```python
from build123d import *

# Parameters (mm, degrees)
SKETCH1_R           = 101.6
BOSS_EXTRUDE1_DEPTH = 25.4
CUT_EXTRUDE1_DEPTH  = 25.4
SKETCH3_R           = 12.7
CUT_EXTRUDE2_DEPTH  = 25.4


with BuildPart() as part:
    # Sketch1 → Boss-Extrude1 (new body)
    with BuildSketch(Plane(origin=(0, 0, 0), x_dir=(1, 0, 0), z_dir=(0, 1, 0))):
        with Locations(Location((0, 0, 0), (0, 0, 270))):
            Circle(SKETCH1_R)
    extrude(amount=BOSS_EXTRUDE1_DEPTH)

    # Sketch2 → Cut-Extrude1 (cut)
    with BuildSketch(Plane(origin=(0, 25.4, 0), x_dir=(1, 0, 0), z_dir=(0, 1, 0))):
        with BuildLine():
            Line((0, 91.44), (16.738974461, 91.44))
            ThreePointArc((16.738974461, 91.44), (20.64808073, 89.604270053), (21.73196517, 85.423814242))
            Line((21.73196517, 85.423814242), (16.01696517, 54.943814242))
            ThreePointArc((16.01696517, 54.943814242), (14.268244513, 51.970893731), (11.023974461, 50.8))
            Line((11.023974461, 50.8), (0, 50.8))
            Line((0, 50.8), (-11.023974461, 50.8))
            ThreePointArc((-11.023974461, 50.8), (-14.268244513, 51.970893731), (-16.01696517, 54.943814242))
            Line((-16.01696517, 54.943814242), (-21.73196517, 85.423814242))
            ThreePointArc((-21.73196517, 85.423814242), (-20.64808073, 89.604270053), (-16.738974461, 91.44))
            Line((-16.738974461, 91.44), (0, 91.44))
        make_face()
        with BuildLine():
            Line((38.26171821, 79.407476156), (23.047495859, 52.38491034))
            ThreePointArc((23.047495859, 52.38491034), (22.476137132, 48.983465131), (24.208756195, 46.001131903))
            Line((24.208756195, 46.001131903), (32.653610572, 38.91505771))
            Line((32.653610572, 38.91505771), (41.098464949, 31.828983518))
            ThreePointArc((41.098464949, 31.828983518), (44.336355977, 30.640563561), (47.586910188, 31.793896828))
            Line((47.586910188, 31.793896828), (71.557020524, 51.469400264))
            ThreePointArc((71.557020524, 51.469400264), (73.413862069, 55.368522696), (71.599297399, 59.287498497))
            Line((71.599297399, 59.287498497), (58.77649903, 70.047103879))
            Line((58.77649903, 70.047103879), (45.953700661, 80.806709261))
            ThreePointArc((45.953700661, 80.806709261), (41.77916706, 81.913183611), (38.26171821, 79.407476156))
        make_face()
        with BuildLine():
            Line((80.352318408, 36.23549746), (51.327777432, 25.314524697))
            ThreePointArc((51.327777432, 25.314524697), (48.703684419, 23.076128807), (48.113940777, 19.677822943))
            Line((48.113940777, 19.677822943), (50.028233853, 8.821327425))
            Line((50.028233853, 8.821327425), (51.942526929, -2.035168092))
            ThreePointArc((51.942526929, -2.035168092), (53.658993735, -5.026826831), (56.890411059, -6.232738262))
            Line((56.890411059, -6.232738262), (87.899750706, -6.568118115))
            ThreePointArc((87.899750706, -6.568118115), (91.828481442, -4.774771782), (92.957513347, -0.606282461))
            Line((92.957513347, -0.606282461), (90.050820935, 15.878389366))
            Line((90.050820935, 15.878389366), (87.144128524, 32.363061192))
            ThreePointArc((87.144128524, 32.363061192), (84.65747826, 35.894008194), (80.352318408, 36.23549746))
        make_face()
        with BuildLine():
            Line((84.845175807, -23.891473209), (55.5912215, -13.600808392))
            ThreePointArc((55.5912215, -13.600808392), (52.142236485, -13.628784649), (49.506077743, -15.852958066))
            Line((49.506077743, -15.852958066), (43.994090512, -25.4))
            Line((43.994090512, -25.4), (38.482103282, -34.947041934))
            ThreePointArc((38.482103282, -34.947041934), (37.873991971, -38.342109081), (39.574256329, -41.34300585))
            Line((39.574256329, -41.34300585), (63.113210637, -61.532341033))
            ThreePointArc((63.113210637, -61.532341033), (67.275533788, -62.683897478), (70.819875692, -60.216377116))
            Line((70.819875692, -60.216377116), (79.189362922, -45.72))
            Line((79.189362922, -45.72), (87.558850152, -31.223622884))
            ThreePointArc((87.558850152, -31.223622884), (87.923614518, -26.920372575), (84.845175807, -23.891473209))
        make_face()
        with BuildLine():
            Line((49.638032496, -72.83935804), (33.8429152, -46.152172078))
            ThreePointArc((33.8429152, -46.152172078), (31.182856603, -43.956638301), (27.733770733, -43.965963811))
            Line((27.733770733, -43.965963811), (17.374623281, -47.736385136))
            Line((17.374623281, -47.736385136), (7.015475828, -51.506806461))
            ThreePointArc((7.015475828, -51.506806461), (4.367328442, -53.716692368), (3.740867244, -57.108421524))
            Line((3.740867244, -57.108421524), (8.795297885, -87.704897725))
            ThreePointArc((8.795297885, -87.704897725), (11.24361619, -91.26253089), (15.544831125, -91.650559689))
            Line((15.544831125, -91.650559689), (31.274321906, -85.925493245))
            Line((31.274321906, -85.925493245), (47.003812686, -80.2004268))
            ThreePointArc((47.003812686, -80.2004268), (50.049314382, -77.138411829), (49.638032496, -72.83935804))
        make_face()
        with BuildLine():
            Line((-8.795297885, -87.704897725), (-3.740867244, -57.108421524))
            ThreePointArc((-3.740867244, -57.108421524), (-4.367328442, -53.716692368), (-7.015475828, -51.506806461))
            Line((-7.015475828, -51.506806461), (-17.374623281, -47.736385136))
            Line((-17.374623281, -47.736385136), (-27.733770733, -43.965963811))
            ThreePointArc((-27.733770733, -43.965963811), (-31.182856603, -43.956638301), (-33.8429152, -46.152172078))
            Line((-33.8429152, -46.152172078), (-49.638032496, -72.83935804))
            ThreePointArc((-49.638032496, -72.83935804), (-50.049314382, -77.138411829), (-47.003812686, -80.2004268))
            Line((-47.003812686, -80.2004268), (-31.274321906, -85.925493245))
            Line((-31.274321906, -85.925493245), (-15.544831125, -91.650559689))
            ThreePointArc((-15.544831125, -91.650559689), (-11.24361619, -91.26253089), (-8.795297885, -87.704897725))
        make_face()
        with BuildLine():
            Line((-63.113210637, -61.532341033), (-39.574256329, -41.34300585))
            ThreePointArc((-39.574256329, -41.34300585), (-37.873991971, -38.342109081), (-38.482103282, -34.947041934))
            Line((-38.482103282, -34.947041934), (-43.994090512, -25.4))
            Line((-43.994090512, -25.4), (-49.506077743, -15.852958066))
            ThreePointArc((-49.506077743, -15.852958066), (-52.142236485, -13.628784649), (-55.5912215, -13.600808392))
            Line((-55.5912215, -13.600808392), (-84.845175807, -23.891473209))
            ThreePointArc((-84.845175807, -23.891473209), (-87.923614518, -26.920372575), (-87.558850152, -31.223622884))
            Line((-87.558850152, -31.223622884), (-79.189362922, -45.72))
            Line((-79.189362922, -45.72), (-70.819875692, -60.216377116))
            ThreePointArc((-70.819875692, -60.216377116), (-67.275533788, -62.683897478), (-63.113210637, -61.532341033))
        make_face()
        with BuildLine():
            Line((-87.899750706, -6.568118115), (-56.890411059, -6.232738262))
            ThreePointArc((-56.890411059, -6.232738262), (-53.658993735, -5.026826831), (-51.942526929, -2.035168092))
            Line((-51.942526929, -2.035168092), (-50.028233853, 8.821327425))
            Line((-50.028233853, 8.821327425), (-48.113940777, 19.677822943))
            ThreePointArc((-48.113940777, 19.677822943), (-48.703684419, 23.076128807), (-51.327777432, 25.314524697))
            Line((-51.327777432, 25.314524697), (-80.352318408, 36.23549746))
            ThreePointArc((-80.352318408, 36.23549746), (-84.65747826, 35.894008194), (-87.144128524, 32.363061192))
            Line((-87.144128524, 32.363061192), (-90.050820935, 15.878389366))
            Line((-90.050820935, 15.878389366), (-92.957513347, -0.606282461))
            ThreePointArc((-92.957513347, -0.606282461), (-91.828481442, -4.774771782), (-87.899750706, -6.568118115))
        make_face()
        with BuildLine():
            Line((-71.557020524, 51.469400264), (-47.586910188, 31.793896828))
            ThreePointArc((-47.586910188, 31.793896828), (-44.336355977, 30.640563561), (-41.098464949, 31.828983518))
            Line((-41.098464949, 31.828983518), (-32.653610572, 38.91505771))
            Line((-32.653610572, 38.91505771), (-24.208756195, 46.001131903))
            ThreePointArc((-24.208756195, 46.001131903), (-22.476137132, 48.983465131), (-23.047495859, 52.38491034))
            Line((-23.047495859, 52.38491034), (-38.26171821, 79.407476156))
            ThreePointArc((-38.26171821, 79.407476156), (-41.77916706, 81.913183611), (-45.953700661, 80.806709261))
            Line((-45.953700661, 80.806709261), (-58.77649903, 70.047103879))
            Line((-58.77649903, 70.047103879), (-71.599297399, 59.287498497))
            ThreePointArc((-71.599297399, 59.287498497), (-73.413862069, 55.368522696), (-71.557020524, 51.469400264))
        make_face()
    extrude(amount=-CUT_EXTRUDE1_DEPTH, mode=Mode.SUBTRACT)

    # Sketch3 → Cut-Extrude2 (cut)
    with BuildSketch(Plane(origin=(0, 25.4, 0), x_dir=(1, 0, 0), z_dir=(0, 1, 0))):
        with Locations(Location((0, 0, 0), (0, 0, 270))):
            Circle(SKETCH3_R)
    extrude(amount=-CUT_EXTRUDE2_DEPTH, mode=Mode.SUBTRACT)


solid = part.part
```
Model file for the job. Use its own axes, mm. Coordinates: 2 decimals unless noted, no trailing zeros. Order: outer loops, then holes, each group sorted by start corner. A loop starts at its lowest first (then second) coordinate and runs counter-clockwise, first axis right, second up. Notation, with made-up numbers: (42.25, 22.5) -> (71.25, 22.5) arc R28 cw to (71.25, 57.5) -> close; hole circle Ø8 at (-26.5, 47.5). An arc over 180 degrees is marked (long way). Return JSON: item names as keys, results as strings.
Item 1: Slice it at B-B (y = 15.5). Count the separate pieces of the cut face and the enclosed holes in it, then the cut area to 3 significant figures.
Model answer:
{"separate pieces": "1", "enclosed holes": "10", "area": "18,200 mm²"}
Item 2: Slice it at A-A (x = 0). Write the cut outline in (y, z).
Model answer:
{"outline": "(0, -101.6) -> (25.4, -101.6) -> (25.4, -91.44) -> (0, -91.44) -> close; (0, -50.8) -> (25.4, -50.8) -> (25.4, -12.7) -> (0, -12.7) -> close; (0, 12.7) -> (25.4, 12.7) -> (25.4, 101.6) -> (0, 101.6) -> close"}
Item 3: Pin check, flat tips, straight feed: P1, Ø12, axis at y = 7.5, z = -80, coming from the +X side; P2, Ø1, axis at x = 77, y = 22.5, coming from the -Z side; P3, Ø2, axis at x = -25, y = 14.5, coming from the +Z side; P4, Ø2, axis at x = 73, z = 20.5, coming from the -Y side. Stop position of each tip, or through.
Model answer:
{"P1": "stops at x = 69.62", "P2": "stops at z = -66.86", "P3": "stops at z = 98.72", "P4": "stops at y = 0"}
Item 4: Wall check: line 1 along X through (y, z) = (16.25, 0); line 2 along X through (y, z) = (8, 24.5); line 3 along X through (y, z) = (19, -10.5). Give the ranges that are in metal, low to high. Write a range as from..to.
Model answer:
{"line 1": "x = -101.6..-92.85, -51.58..-12.7, 12.7..51.58, 92.85..101.6", "line 2": "x = -98.6..-86.04, -44.51..44.51, 86.04..98.6", "line 3": "x = -101.06..-91, -49.73..-7.14, 7.14..49.73, 91..101.06"}
Item 5: Slice it at C-C (x = 77.5). Write the cut outline in (y, z).
Model answer:
{"outline": "(0, -65.7) -> (25.4, -65.7) -> (25.4, -35.16) -> (0, -35.16) -> close; (0, 6.46) -> (25.4, 6.46) -> (25.4, 21.31) -> (0, 21.31) -> close; (0, 48.65) -> (25.4, 48.65) -> (25.4, 65.7) -> (0, 65.7) -> close"}
